```python
from build123d import *

# Parameters (mm, degrees)
SKETCH1_W           = 254
SKETCH1_H           = 25.4
BOSS_EXTRUDE1_DEPTH = 6.35
CUT_EXTRUDE1_DEPTH  = 128.791284914
CUT_EXTRUDE2_DEPTH  = 3.81


with BuildPart() as part:
    # Sketch1 → Boss-Extrude1 (new body)
    with BuildSketch(Plane(origin=(0, 0, 0), x_dir=(1, 0, 0), z_dir=(0, 1, 0))):
        Rectangle(SKETCH1_W, SKETCH1_H)
    extrude(amount=BOSS_EXTRUDE1_DEPTH)

    # Sketch2 → Cut-Extrude1 (cut, through all)
    with BuildSketch(Plane(origin=(0, 6.35, 0), x_dir=(1, 0, 0), z_dir=(0, 1, 0))):
        with BuildLine():
            Line((-114.3, 3.3782), (114.3, 3.3782))
            ThreePointArc((114.3, 3.3782), (117.6782, 0), (114.3, -3.3782))
            Line((114.3, -3.3782), (-114.3, -3.3782))
            ThreePointArc((-114.3, -3.3782), (-117.6782, 0), (-114.3, 3.3782))
        make_face()
    extrude(amount=-CUT_EXTRUDE1_DEPTH, mode=Mode.SUBTRACT)

    # Sketch3 → Cut-Extrude2 (cut)
    with BuildSketch(Plane.XZ):
        with BuildLine():
            Line((-114.3, 6.477), (114.3, 6.477))
            ThreePointArc((114.3, 6.477), (120.777, 0), (114.3, -6.477))
            Line((114.3, -6.477), (-114.3, -6.477))
            ThreePointArc((-114.3, -6.477), (-120.777, 0), (-114.3, 6.477))
        make_face()
    extrude(amount=-CUT_EXTRUDE2_DEPTH, mode=Mode.SUBTRACT)


solid = part.part
```
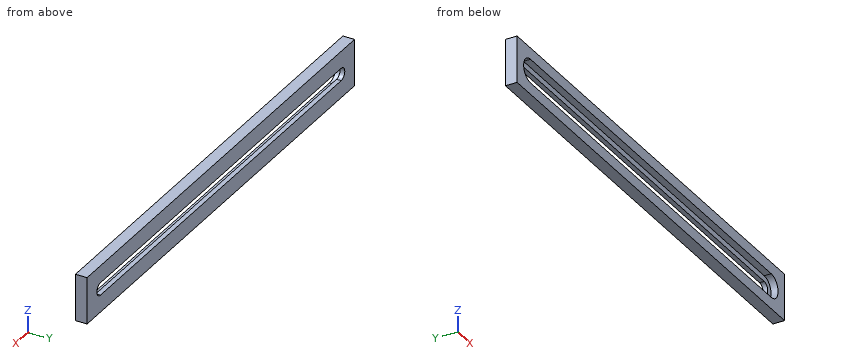
The listing builds one solid part. Answer for the finished solid, in the listing's coordinates (mm). Coordinates: 2 decimals unless noted, no trailing zeros. Order: outer loops, then holes, each group sorted by start corner. A loop starts at its lowest first (then second) coordinate and runs counter-clockwise, first axis right, second up. Notation, with made-up numbers: M 74.25,43 L 96.25,43 A28 cw 96.25,78 Z; hole C -18.75,-17 d1. An arc over 180 degrees is marked long. Answer as a JSON object with one key per item and string values. Group by question number.
1. Section C-C on y = 5.25 is taken. Write down the section's boundary in (x, z), then the cut area to 3 significant figures.
2. A flat-ended cylindrical pin translates along its axis: P1, Ø5, axis at x = 58.5, z = 0, coming from the +Y side. Find the tip coordinate at first contact, or state that the pin passes through.
3. Section B-B on z = 0 is taken. Write down the section's boundary in (x, y).
4. Straight lines are drawn through the part: line 1 (Z direction, x = -51.5, y = 6.25); line 2 (Z direction, x = 5, y = 1.75); line 3 (X direction, y = 2, z = -4.5). For each, find the intervals that lie inside material, in ascending order.
5. Section A-A on x = 100 is taken. Write down the section's boundary in (y, z), then the cut area to 3 significant figures.
Values follow:
{
 "1": {"outline": "M -127,-12.7 L 127,-12.7 L 127,12.7 L -127,12.7 Z; hole M -114.3,-3.38 L 114.3,-3.38 A3.38 ccw 114.3,3.38 L -114.3,3.38 A3.38 ccw Z", "area": "4,870 mm2"},
 "2": {"P1": "through"},
 "3": {"outline": "M -127,0 L -120.78,0 L -120.78,3.81 L -117.68,3.81 L -117.68,6.35 L -127,6.35 Z; M 117.68,3.81 L 120.78,3.81 L 120.78,0 L 127,0 L 127,6.35 L 117.68,6.35 Z"},
 "4": {"line 1": "-12.7 to -3.38, 3.38 to 12.7", "line 2": "-12.7 to -6.48, 6.48 to 12.7", "line 3": "-127 to -118.96, 118.96 to 127"},
 "5": {"outline": "M 0,-12.7 L 6.35,-12.7 L 6.35,-3.38 L 3.81,-3.38 L 3.81,-6.48 L 0,-6.48 Z; M 0,6.48 L 3.81,6.48 L 3.81,3.38 L 6.35,3.38 L 6.35,12.7 L 0,12.7 Z", "area": "94.8 mm2"}
}
